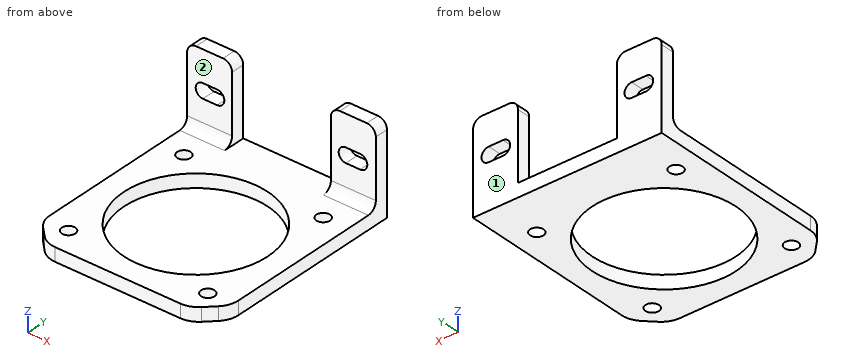
from build123d import *

# Parameters (mm, degrees)
F0_R     = 1.5
F0_R_2   = 16
F1_DEPTH = 3
F0_W     = 42
F0_H     = 3
F2_DEPTH = 20
F4_DEPTH = 25
F3_W     = 22
F3_H     = 17
F5_DEPTH = 25
F6_R     = 2
F7_R     = 5


with BuildPart() as f1:
    # F0 (on Top) → F1 (new body)
    with BuildSketch(Plane.XY):
        Polygon((-96.9759252071, -84.7722164392), (-91.9759252071, -79.7722164392), (-91.9759252071, -47.7722164392), (-91.9759252071, -42.7722164392), (-91.9759252071, -40.7722164392), (-133.9759252071, -40.7722164392), (-133.9759252071, -42.7722164392), (-133.9759252071, -47.7722164392), (-133.9759252071, -79.7722164392), (-128.9759252071, -84.7722164392), align=None)
        with Locations((-128.4759252071, -79.2722164392)):
            Circle(F0_R, mode=Mode.SUBTRACT)
        with Locations((-97.4759252071, -79.2722164392)):
            Circle(F0_R, mode=Mode.SUBTRACT)
        with Locations((-112.9759252071, -63.7722164392)):
            Circle(F0_R_2, mode=Mode.SUBTRACT)
        with Locations((-128.4759252071, -48.2722164392)):
            Circle(F0_R, mode=Mode.SUBTRACT)
        with Locations((-97.4759252071, -48.2722164392)):
            Circle(F0_R, mode=Mode.SUBTRACT)
    extrude(amount=F1_DEPTH)

    # F0 (on Top) → F2 (join)
    with BuildSketch(Plane.XY):
        with Locations((-112.9759252071, -39.2722164392)):
            Rectangle(F0_W, F0_H)
    extrude(amount=F2_DEPTH)

    # F3 (on face) → F4 (cut)
    with BuildSketch(Plane.XZ.offset(40.7722164392)):
        with BuildLine():
            ThreePointArc((-95.4759252071, 9.9), (-93.8759252071, 11.5), (-95.4759252071, 13.1))
            Line((-95.4759252071, 13.1), (-98.6511558294, 13.1))
            ThreePointArc((-98.6511558294, 13.1), (-100.2511558294, 11.5), (-98.6511558294, 9.9))
            Line((-98.6511558294, 9.9), (-95.4759252071, 9.9))
        make_face()
        with BuildLine():
            Line((-127.3006945848, 13.1), (-130.4759252071, 13.1))
            ThreePointArc((-130.4759252071, 13.1), (-132.0759252071, 11.5), (-130.4759252071, 9.9))
            Line((-130.4759252071, 9.9), (-127.3006945848, 9.9))
            ThreePointArc((-127.3006945848, 9.9), (-125.7006945848, 11.5), (-127.3006945848, 13.1))
        make_face()
    extrude(amount=-F4_DEPTH, mode=Mode.SUBTRACT)

    # F3 (on face) → F5 (cut)
    with BuildSketch(Plane.XZ.offset(40.7722164392)):
        with Locations((-112.9759252071, 11.5)):
            Rectangle(F3_W, F3_H)
    extrude(amount=-F5_DEPTH, mode=Mode.SUBTRACT)

    # F6
    f6_edges = [f1.edges().sort_by_distance(p)[0] for p in [
        (-96.975925, -40.772216, 3),
        (-128.975925, -40.772216, 3),
        (-91.975925, -39.272216, 20),
        (-101.975925, -39.272216, 20),
        (-123.975925, -39.272216, 20),
        (-133.975925, -39.272216, 20),
    ]]
    fillet(f6_edges, radius=F6_R)

    # F7
    f7_edges = [f1.edges().sort_by_distance(p)[0] for p in [
        (-133.975925, -79.772216, 1.5),
        (-128.975925, -84.772216, 1.5),
        (-96.975925, -84.772216, 1.5),
        (-91.975925, -79.772216, 1.5),
    ]]
    fillet(f7_edges, radius=F7_R)


solid = f1.part
Can you work these out from the model? Positions are in its coordinate system, mm. Face numbers are marked on the shaded views. A direction names the side the tool comes from. Coordinates: 2 decimals unless noted, no trailing zeros. Write each loop counter-clockwise with the first axis right and the second up, starting at its lowest first coordinate (ties: lowest second). Pieces come first, ordered by that corner, then holes. Notation, with made-up numbers: (-21.5, -17.75) - (-6.5, -17.75) arc R22 cw to (-6.5, 1.25) - close; hole circle Ø5 at (-11.5, 9). An arc over 180 degrees is marked (long way). Return JSON: item names as keys, results as strings. Group by question number.
Item 1: If we section it at A-A (z = 15.75): Write out the boundary of the cut face in (x, y), then the cut area to 3 significant figures.
Item 2: Please list where these lines run through material, in increasing order: probe 1 along Z at (x, y) = (-112.5, -46.5); probe 2 along Y at (x, z) = (-101, 16.5); probe 3 along Y at (x, z) = (-121, 1.75).
Item 3: If we section it at C-C (z = 11.5): Write out the boundary of the cut face in (x, y).
Item 4: Which directions (+Z, -Z, +X, -X, +Y, -Y) give clear straight access to the entire face, cutting with the end or side of a thin tool? Please do the marked faces 1 and 2.
Item 5: I'm going to push flat-ended pins straight in: pin 1 Ø10 at (x, y) = (-127.5, -58) entering from +Z; pin 2 Ø19 at (x, y) = (-112.98, -63.77) entering from +Z; pin 3 Ø3 at (x, z) = (-95, 9.5) entering from -Y. Where does each tip first touch, or does it pass through?
Item 6: If we section it at D-D (x = -101): Write out the boundary of the cut face in (y, z).
Item 7: If we section it at B-B (x = -113): Write out the boundary of the cut face in (y, z).
Return value:
{
 "1": {"outline": "(-133.98, -40.77) - (-123.98, -40.77) - (-123.98, -37.77) - (-133.98, -37.77) - close; (-101.98, -40.77) - (-91.98, -40.77) - (-91.98, -37.77) - (-101.98, -37.77) - close", "area": "60.0 mm^2"},
 "2": {"probe 1": "z = 0 to 3", "probe 2": "y = -40.77 to -37.77", "probe 3": "y = -84.77 to -77.61, -49.93 to -37.77"},
 "3": {"outline": "(-133.98, -40.77) - (-132.08, -40.77) - (-132.08, -37.77) - (-133.98, -37.77) - close; (-125.7, -40.77) - (-123.98, -40.77) - (-123.98, -37.77) - (-125.7, -37.77) - close; (-101.98, -40.77) - (-100.25, -40.77) - (-100.25, -37.77) - (-101.98, -37.77) - close; (-93.88, -40.77) - (-91.98, -40.77) - (-91.98, -37.77) - (-93.88, -37.77) - close"},
 "4": {"face 1": "+Z, -Z, +X, -X, +Y", "face 2": "+Z, +X, -X, -Y"},
 "5": {"pin 1": "stops at z = 3", "pin 2": "passes through", "pin 3": "stops at y = -40.77"},
 "6": {"outline": "(-84.77, 0) - (-74.38, 0) - (-74.38, 3) - (-84.77, 3) - close; (-53.16, 0) - (-37.77, 0) - (-37.77, 19.72) - (-40.77, 19.72) - (-40.77, 5) arc R2 cw to (-42.77, 3) - (-53.16, 3) - close"},
 "7": {"outline": "(-84.77, 0) - (-79.77, 0) - (-79.77, 3) - (-84.77, 3) - close; (-47.77, 0) - (-37.77, 0) - (-37.77, 3) - (-47.77, 3) - close"}
}
